```python
from build123d import *

# Parameters (mm, degrees)
BOSS_EXTRUDE1_DEPTH = 381
SKETCH5_W           = 63.5
SKETCH5_H           = 25.4
BOSS_EXTRUDE4_DEPTH = 101.6
SKETCH6_R           = 19.05
CUT_EXTRUDE3_DEPTH  = 25.4
FILLET3_R           = 50.8
FILLET4_R           = 12.7
FILLET5_R           = 50.8
SKETCH7_W           = 63.5
SKETCH7_H           = 25.4
BOSS_EXTRUDE5_DEPTH = 101.6
SKETCH8_R           = 19.05
CUT_EXTRUDE4_DEPTH  = 25.4


with BuildPart() as part:
    # Sketch1 → Boss-Extrude1 (new body)
    with BuildSketch(Plane.XY):
        Polygon((0, 7.775510204), (0, 0), (6.220408163, 0), (1828.8, 0), (2133.6, 175.976362049), (2133.6, 252.176362049), (1828.8, 76.2), (76.2, 76.2), (76.2, 609.6), (0, 609.6), align=None)
    extrude(amount=BOSS_EXTRUDE1_DEPTH)

    # Sketch5 → Boss-Extrude4 (add)
    with BuildSketch(Plane.ZY):
        with Locations((190.5, 63.5)):
            Rectangle(SKETCH5_W, SKETCH5_H)
    extrude(amount=BOSS_EXTRUDE4_DEPTH)

    # Sketch6 → Cut-Extrude3 (cut)
    with BuildSketch(Plane(origin=(0, 76.2, 0), x_dir=(1, 0, 0), z_dir=(0, 1, 0))):
        with Locations(Location((-63.5, -190.5, 0), (0, 0, 270))):
            Circle(SKETCH6_R)
    extrude(amount=-CUT_EXTRUDE3_DEPTH, mode=Mode.SUBTRACT)

    # Fillet3
    fillet3_edges = [part.edges().sort_by_distance(p)[0] for p in [
        (1828.8, 0, 190.5),
    ]]
    fillet(fillet3_edges, radius=FILLET3_R)

    # Fillet4
    fillet4_edges = [part.edges().sort_by_distance(p)[0] for p in [
        (2133.6, 252.176362049, 190.5),
    ]]
    fillet(fillet4_edges, radius=FILLET4_R)

    # Fillet5
    fillet5_edges = [part.edges().sort_by_distance(p)[0] for p in [
        (0, 0, 190.5),
    ]]
    fillet(fillet5_edges, radius=FILLET5_R - 0.0001)  # a hair under: the kernel refuses the full size

    # Sketch7 → Boss-Extrude5 (add)
    with BuildSketch(Plane(origin=(2133.6, 0, 0), x_dir=(0, 0, -1), z_dir=(1, 0, 0))):
        with Locations((-190.5, 201.376362049)):
            Rectangle(SKETCH7_W, SKETCH7_H)
    extrude(amount=BOSS_EXTRUDE5_DEPTH)

    # Sketch8 → Cut-Extrude4 (cut)
    with BuildSketch(Plane(origin=(0, 214.076362049, 0), x_dir=(1, 0, 0), z_dir=(0, 1, 0))):
        with Locations(Location((2203.45, -190.5, 0), (0, 0, 180))):
            Circle(SKETCH8_R)
    extrude(amount=-CUT_EXTRUDE4_DEPTH, mode=Mode.SUBTRACT)


solid = part.part
```
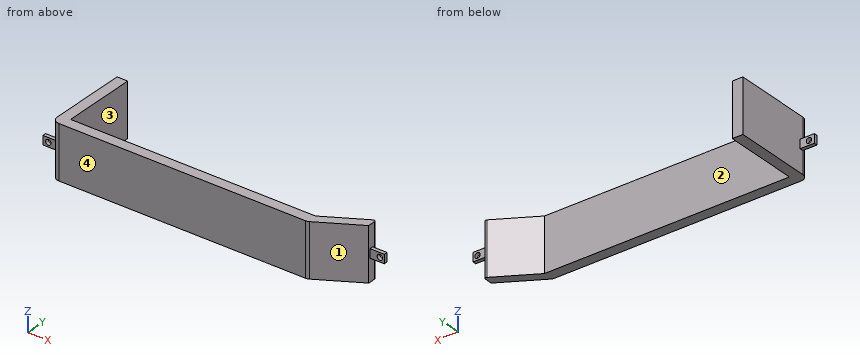
Can you work these out from the model? Positions are in its coordinate system, mm. Face numbers are marked on the shaded views. Round coordinates to 2 decimals unless told otherwise and drop trailing zeros. Loops run counter-clockwise (first coordinate to the right, second up) from the corner with the lowest first, then second, coordinate; pieces in that order, holes last. Notation, with made-up numbers: M 2,73 L 29,73 A19 cw 29,103 Z; hole C 14.5,78 d2. An arc over 180 degrees is marked long. Write item = value, one per line. Start each with the question number.
(1) Suppose I cut it at C-C on y = 380. Write out the boundary of the cut face in (x, z), plus the area to 3 significant figures.
(2) Suppose I cut it at B-B on z = 339. Write out the boundary of the cut face in (x, y).
(3) If we mould it in two halves opening along X, with no side actions, what happens to the marked faces 1, 2, 3 and 4? For each: released by +X, released by -X, zero draft, split by the parting line, or undercut.
(4) Suppose I cut it at A-A on y = 122.5. Write out the boundary of the cut face in (x, z).
(5) I'm going to push flat-ended pins straight in: P1, Ø6, axis at y = 338.5, z = 281, coming from the -X side; P2, Ø16.5, axis at y = 198.5, z = 285.5, coming from the +X side; P3, Ø8, axis at x = 1762.5, z = 300.5, coming from the +Y side; P4, Ø23, axis at x = -63.5, z = 190.5, coming from the -Y side. Where does each tip first touch, or does it pass through?
(6) I need wall thicknesses on line 1 along Z through (x, y) = (2203.45, 194); line 2 along Y through (x, z) = (950.5, 41); line 3 along X through (y, z) = (70, 190.5). Which ranges of each line are inside material? Lowest first, please.
Answer block:
q1.outline = M 0,0 L 76.2,0 L 76.2,381 L 0,381 Z
q1.area = 29,000 mm²
q2.outline = M 0,50.8 A50.8 ccw 50.8,0 L 1815.19,0 A50.8 ccw 1840.59,6.81 L 2133.6,175.98 L 2133.6,230.18 A12.7 ccw 2114.55,241.18 L 1828.8,76.2 L 76.2,76.2 L 76.2,609.6 L 0,609.6 Z
q3.face_1 = released by +X
q3.face_2 = undercut
q3.face_3 = undercut
q3.face_4 = zero draft
q4.outline = M 0,0 L 76.2,0 L 76.2,381 L 0,381 Z; M 1908.99,0 L 2040.98,0 L 2040.98,381 L 1908.99,381 Z
q5.P1 = 0
q5.P2 = 2133.6
q5.P3 = 76.2
q5.P4 = through
q6.line_1 = 158.75 to 171.45, 209.55 to 222.25
q6.line_2 = 0 to 76.2
q6.line_3 = -101.6 to -82.55, -44.45 to 1950.04
